```python
from build123d import *

# Parameters (mm, degrees)
F0_W     = 12.7
F0_H     = 2.54
F3_W     = 2.54
F3_H     = 2.54
F4_DEPTH = 12.7


with BuildPart() as f2:
    # F2: sweep along a path in F1
    with BuildLine(Plane.XZ) as f2_path:
        Line((0, 0), (177.8, 0))
        Line((177.8, 0), (177.8, -12.7))
        Line((177.8, -12.7), (0, -12.7))
        Line((0, -12.7), (0, 0))
    # F0 (on Right) → F2 (sweep)
    with BuildSketch(Plane.YZ):
        with Locations((6.35, -1.27)):
            Rectangle(F0_W, F0_H)
    sweep(path=f2_path.line, transition=Transition.RIGHT)

    # F3 (on face) → F4 (join)
    with BuildSketch(Plane.XY):
        with Locations((45.72, 6.35)):
            Rectangle(F3_W, F3_H)
        with Locations((90.17, 6.35)):
            Rectangle(F3_W, F3_H)
        with Locations((134.62, 6.35)):
            Rectangle(F3_W, F3_H)
    extrude(amount=-F4_DEPTH)


solid = f2.part
```
CAD build for the part. Positions are in the model's coordinates, mm. A direction names the side the tool comes from. Round coordinates to 2 decimals unless told otherwise and drop trailing zeros. Order: outer loops, then holes, each group sorted by start corner. A loop starts at its lowest first (then second) coordinate and runs counter-clockwise, first axis right, second up. Notation, with made-up numbers: (62.25, 72.25) - (114.25, 72.25) arc R26 ccw to (114.25, 88.25) - close; hole circle Ø8 at (-7.75, 13.5). An arc over 180 degrees is marked (long way). Answer in a Markdown table with one row per item. Add a question column.
(1) Drop flat-ended pins along their axis: pin 1 Ø0.8 at (x, z) = (134.5, -8) entering from -Y; pin 2 Ø3 at (x, z) = (45.5, -5) entering from +Y. Give the stop position or say it passes through.
(2) 3-axis set-ups, long thin cutter, end or side, ignore diameter. For faces 1 (the face through (88, 6, -12.7)), 2 (the face through (175.26, 6, -6)): which of +Z, -Z, +X, -X, +Y, -Y reach the whole face in a straight line?
(3) Band-saw the part on A-A on x = 151. List the corners of the cut face in (y, z), and give its area (3 significant figures).
(4) Probe L1, parallel to X at y = 5.5, z = -3.75; L2, parallel to X at y = 5, z = -9; L3, parallel to Z at x = 53.5, y = 2.5. List the from-to ranges inside material, lowest first. Write a range as [from, to].
(5) Band-saw the part on B-B on z = -6. List the corners of the cut face in (x, y).
(6) Band-saw the part on C-C on y = 1.5. List the corners of the cut face in (x, z), and give its area (3 significant figures).
(7) Mould opens along Z. For faces 3 (the face through (90, 8, -2.54)), 4 (the face through (90, 0, -2)), 5 (the face through (88, 6, 0)) say: +Z half, -Z half, draft (parallel to the pull), parting line (faces both ways), or undercut.
Data:
| question | item | result |
|---|---|---|
| 1 | pin 1 | stops at y = 5.08 |
| 1 | pin 2 | stops at y = 7.62 |
| 2 | face 1 | -Z, +X, -X, +Y, -Y |
| 2 | face 2 | +Y, -Y |
| 3 | outline | (0, -12.7) - (12.7, -12.7) - (12.7, -10.16) - (0, -10.16) - close; (0, -2.54) - (12.7, -2.54) - (12.7, 0) - (0, 0) - close |
| 3 | area | 64.5 mm^2 |
| 4 | L1 | x = [0, 2.54], [44.45, 46.99], [88.9, 91.44], [133.35, 135.89], [175.26, 177.8] |
| 4 | L2 | x = [0, 2.54], [175.26, 177.8] |
| 4 | L3 | z = [-12.7, -10.16], [-2.54, 0] |
| 5 | outline | (0, 0) - (2.54, 0) - (2.54, 12.7) - (0, 12.7) - close; (44.45, 5.08) - (46.99, 5.08) - (46.99, 7.62) - (44.45, 7.62) - close; (88.9, 5.08) - (91.44, 5.08) - (91.44, 7.62) - (88.9, 7.62) - close; (133.35, 5.08) - (135.89, 5.08) - (135.89, 7.62) - (133.35, 7.62) - close; (175.26, 0) - (177.8, 0) - (177.8, 12.7) - (175.26, 12.7) - close |
| 6 | outline | (0, -12.7) - (177.8, -12.7) - (177.8, 0) - (0, 0) - close; hole (2.54, -10.16) - (175.26, -10.16) - (175.26, -2.54) - (2.54, -2.54) - close |
| 6 | area | 942 mm^2 |
| 7 | face 3 | undercut |
| 7 | face 4 | draft |
| 7 | face 5 | +Z half |
